Model file for the job. Use its own axes, mm. Face numbers are marked on the shaded views. A direction names the side the tool comes from. Give positions to 0.01 mm unless a question says otherwise; leave off trailing zeros. Order: outer loops, then holes, each group sorted by start corner. A loop starts at its lowest first (then second) coordinate and runs counter-clockwise, first axis right, second up. Notation, with made-up numbers: (64.25, 8.5) -> (90.25, 8.5) arc R4 cw to (90.25, 15.5) -> close; hole circle Ø7 at (9.5, 27). An arc over 180 degrees is marked (long way). Answer in a Markdown table with one row per item. Add a question column.
Solid Edge part; units mm, degrees
sketch "Sketch1" plane through (0, 0, 0) normal (1, 0, 0) x (0, 1, 0)
  line L0 (4, 5.4) -> (4, 0.9)
  line L1 (4, 0.9) -> (3.2143, 0.9)
  line L2 (3.2143, 0.9) -> (3.2143, 5.4)
  line L3 (3.2143, 5.4) -> (1.4, 5.4)
  line L4 (1.4, 5.4) -> (1.4, 0)
  line L5 (1.4, 0) -> (0, 0)
  line L6 (0, 0) -> (0, 6)
  line L7 (0, 6) -> (1.4, 6)
  line L8 (1.4, 6) -> (4, 6)
  line L9 (4, 6) -> (4, 5.4)
revolve "RevolvedProtrusion1" add sketch "Sketch1" angle 360 about axis through (0, 0, 0) along (0, 0, 1)
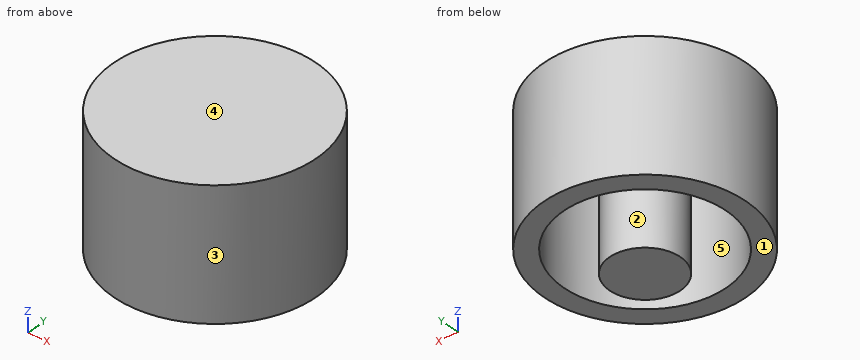
Item 1: Wall check: line 1 (Y direction, x = 0, z = 4.35); line 2 (Y direction, x = 1, z = 2.3). Give the ranges that are in metal, low to high.
Item 2: Saw through at D-D on y = 2. List the corners of the cut face in (x, z).
Item 3: Which spindle directions (+Z, -Z, +X, -X, +Y, -Y) get a long thin tool onto all of the face, cutting with end or side? Do the marked faces 4 and 5. Say none if no direction does.
Item 4: Pin check, flat tips, straight feed: pin 1 Ø2 at (y, z) = (1.5, 1) entering from -X; pin 2 Ø1 at (x, y) = (-0.5, -2.5) entering from -Z; pin 3 Ø1.5 at (x, y) = (2, -3) entering from -Z. Stop position of each tip, or through.
Item 5: Saw through at A-A on z = 1.6. List the corners of the cut face in (x, y).
Item 6: Two-plate mould, pull along Y, no slides. Class the marked faces 1, 2 and 3: pulls with the +Y half, pulls with the -Y half, needs draft (parallel to the pull), parting line crosses it, or undercut.
Item 7: Saw through at B-B on y = 0. List the corners of the cut face in (x, z), plus the area to 3 significant figures.
Evaluation:
| question | item | result |
|---|---|---|
| 1 | line 1 | y = -4 to -3.21, -1.4 to 1.4, 3.21 to 4 |
| 1 | line 2 | y = -3.87 to -3.05, -0.98 to 0.98, 3.05 to 3.87 |
| 2 | outline | (-3.46, 0.9) -> (-2.52, 0.9) -> (-2.52, 5.4) -> (2.52, 5.4) -> (2.52, 0.9) -> (3.46, 0.9) -> (3.46, 6) -> (-3.46, 6) -> close |
| 3 | face 4 | +Z, +X, -X, +Y, -Y |
| 3 | face 5 | -Z |
| 4 | pin 1 | stops at x = -3.97 |
| 4 | pin 2 | stops at z = 5.4 |
| 4 | pin 3 | stops at z = 0.9 |
| 5 | outline | circle Ø8 at (0, 0); circle Ø2.8 at (0, 0); hole circle Ø6.43 at (0, 0) |
| 6 | face 1 | needs draft |
| 6 | face 2 | undercut |
| 6 | face 3 | parting line crosses it |
| 7 | outline | (-4, 0.9) -> (-3.21, 0.9) -> (-3.21, 5.4) -> (-1.4, 5.4) -> (-1.4, 0) -> (1.4, 0) -> (1.4, 5.4) -> (3.21, 5.4) -> (3.21, 0.9) -> (4, 0.9) -> (4, 6) -> (-4, 6) -> close |
| 7 | area | 27.0 mm2 |
